Could you check a few things on this model? Use its own coordinates, in mm. A direction names the side the tool comes from. Give positions to 0.01 mm unless a question says otherwise; leave off trailing zeros. Loops run counter-clockwise (first coordinate to the right, second up) from the corner with the lowest first, then second, coordinate; pieces in that order, holes last. Notation, with made-up numbers: M 4,38 L 8,38 A5 ccw 8,43 Z; hole C 8.5,52.5 d1. An arc over 180 degrees is marked long. Use CSV: the item, a comma, the result in double quotes.
```python
from build123d import *

# Parameters (mm, degrees)
SKETCH1_W            = 15.875
SKETCH1_H            = 15.875
BASE_EXTRUDE_DEPTH   = 3.175
SKETCH2_R            = 2.4384
BOSS_EXTRUDE1_DEPTH  = 1.905
LPATTERN4_COUNT      = 2
LPATTERN4_PITCH      = 7.9375
LPATTERN4_COUNT_DIR2 = 2
LPATTERN4_PITCH_DIR2 = 7.9375
SHELL1_T             = -1.5875
SKETCH3_R            = 3.2004
SKETCH3_R_2          = 2.4384
INSDOT_DEPTH         = 1.5875
FILLET1_R            = 0.254


with BuildPart() as part:
    # Sketch1 → Base-Extrude (new body)
    with BuildSketch(Plane(origin=(0, 0, 0), x_dir=(1, 0, 0), z_dir=(0, 1, 0))):
        Rectangle(SKETCH1_W, SKETCH1_H)
    extrude(amount=BASE_EXTRUDE_DEPTH)

    # Sketch2 → Boss-Extrude1 (add)
    with BuildSketch(Plane(origin=(0, 3.175, 0), x_dir=(-1, 0, 0), z_dir=(0, 1, 0))):
        with Locations(Location((3.96875, 3.96875, 0), (0, 0, 270))):
            Circle(SKETCH2_R)
    boss_extrude1 = extrude(amount=BOSS_EXTRUDE1_DEPTH)

    # LPattern4: Boss-Extrude1 2 × 2
    with Locations(*[(i * LPATTERN4_PITCH, 0, -j * LPATTERN4_PITCH_DIR2) for i in range(LPATTERN4_COUNT) for j in range(LPATTERN4_COUNT_DIR2) if (i, j) != (0, 0)]):
        add(boss_extrude1)

    # Shell1
    shell1_openings = [part.faces().sort_by_distance(p)[0] for p in [
        (0, 0, 0),
    ]]
    offset(amount=SHELL1_T, openings=shell1_openings, kind=Kind.INTERSECTION)

    # Sketch3 → InsDot (add)
    with BuildSketch(Plane.XZ.offset(-1.5875)):
        Circle(SKETCH3_R)
        Circle(SKETCH3_R_2, mode=Mode.SUBTRACT)
    extrude(amount=INSDOT_DEPTH)

    # Fillet1
    fillet1_edges = [part.edges().sort_by_distance(p)[0] for p in [
        (7.9375, 3.175, 0),
        (0, 3.175, -7.9375),
        (-7.9375, 3.175, 0),
        (0, 3.175, 7.9375),
    ]]
    fillet(fillet1_edges, radius=FILLET1_R)


solid = part.part
```
1. If we mould it in two halves opening along X, with no side actions, what happens to faces 1 (the face through (4, 5.08, 4)), 2 (the face through (4, 3.492, 4)), 3 (the face through (7.938, 1, 0)), 4 (the face through (0, 1.588, 0))? For each: +X half, -X half, draft (parallel to the pull), parting line (faces both ways), or undercut.
Outcome:
face 1,"draft"
face 2,"undercut"
face 3,"+X half"
face 4,"undercut"
2. I'm going to push flat-ended pins straight in: pin 1 Ø4.5 at (x, z) = (0, 0) entering from +Y (3 decimals); pin 2 Ø1 at (x, z) = (0, -3) entering from -Y; pin 3 Ø2 at (x, z) = (-3.97, 3.97) entering from -Y; pin 4 Ø1.4 at (x, z) = (-4, 4) entering from -Y. Where does each tip first touch, or does it pass through?
Outcome:
pin 1,"y = 3.175"
pin 2,"y = 0"
pin 3,"y = 1.59"
pin 4,"y = 3.49"
3. I want a section at B-B, the plane y = 1.85. List the corners of the cut face in (x, z) for me.
Outcome:
outline,"M -7.94,-7.94 L 7.94,-7.94 L 7.94,7.94 L -7.94,7.94 Z; hole C -3.97,-3.97 d1.7; hole C -3.97,3.97 d1.7; hole C 3.97,-3.97 d1.7; hole C 3.97,3.97 d1.7"
4. Which directions (+Z, -Z, +X, -X, +Y, -Y) give clear straight access to the entire face, cutting with the end or side of a thin tool? Please do faces 5 (the face through (-7, 0, 0)), 6 (the face through (3.862, 4.114, 6.405)), 7 (the face through (4.49, 2.53, 4.64)).
Outcome:
face 5,"+Z, -Z, +X, -X, -Y"
face 6,"+Y"
face 7,"-Y"
5. Please list where these lines run through material, in increasing order: line 1 (Z direction, x = -4, y = 4.8); line 2 (X direction, y = 0.5, z = 4.25).
Outcome:
line 1,"-6.41 to -1.53, 1.53 to 6.41"
line 2,"-7.94 to -6.35, 6.35 to 7.94"
6. I want a section at D-D, the plane y = 4.4. List the corners of the cut face in (x, z) for me.
Outcome:
outline,"C -3.97,-3.97 d4.88; C -3.97,3.97 d4.88; C 3.97,-3.97 d4.88; C 3.97,3.97 d4.88"
